Design review of the part built by this model. Coordinates are the model's own, in mm. A direction names the side the tool comes from. Give positions to 0.01 mm unless a question says otherwise; leave off trailing zeros. Write each loop counter-clockwise with the first axis right and the second up, starting at its lowest first coordinate (ties: lowest second). Pieces come first, ordered by that corner, then holes. Notation, with made-up numbers: M 76.25,27 L 118.25,27 A11 ccw 118.25,36 Z; hole C 32,47.25 d5. An arc over 180 degrees is marked long. Answer in a Markdown table with one row per item.
Autodesk Inventor part; units mm, degrees
ref_plane "YZ Plane" through (0, 0, 0) normal (1, 0, 0) x (0, 1, 0)
ref_plane "XZ Plane" through (0, 0, 0) normal (0, 1, 0) x (-1, 0, 0)
ref_plane "XY Plane" through (0, 0, 0) normal (0, 0, 1) x (1, 0, 0)
sketch "スケッチ1" plane through (0, 0, 0) normal (0, 1, 0) x (-1, 0, 0)
  line L0 (0, 0) -> (0, 28.5) construction
  line L1 (0, 30) -> (-7.1789, 30)
  line L2 (-8.2396, 29.5607) -> (-18.0607, 19.7396)
  line L3 (-18.5, 18.6789) -> (-18.5, 0)
  line L4 (-18.5, 0) -> (-17, 0)
  line L5 (-17, 0) -> (-17, 18.6789)
  line L6 (-17, 18.6789) -> (-7.1789, 28.5)
  line L7 (-7.1789, 28.5) -> (0, 28.5)
  line L8 (0, 28.5) -> (0, 30)
  line L9 (0, 0) -> (-17, 0) construction
  line L10 (0, 14.25) -> (-10.7145, 24.9645) construction
  arc A0 (-7.1789, 30) -> (-8.2396, 29.5607) centre (-7.1789, 28.5) ccw
  arc A1 (-18.0607, 19.7396) -> (-18.5, 18.6789) centre (-17, 18.6789) ccw
  dimension "d0" = 28.5
  dimension "d1" = 1.5
  dimension "d2" = 1.5
  dimension "d3" = 135
  dimension "d4" = 1.5
  dimension "d5" = 34
  dimension "d7" = 5
  dimension "d8" = 1.5
extrude "押し出し1" add sketch "スケッチ1" against normal blind 15
sketch "スケッチ2" plane through (17, 0, 0) normal (-1, 0, 0) x (0, 0, 1)
  circle A0 centre (3.25, 4.25) radius 1.3
  arc A1 (4.8202, 7.0955) -> (0, 4.25) centre (3.25, 4.25) ccw
  line L0 (0, 4.25) -> (0, 0)
  line L1 (4.8202, 7.0955) -> (17.6789, 0)
  line L2 (18.6789, 0) -> (0, 0) construction
  line L3 (0, 0) -> (0, -15) construction
  line L4 (0, 0) -> (17.6789, 0)
  line L5 (18.6789, 0) -> (18.6789, -15)
  dimension "d11" = 2.6
  dimension "d12" = 4.25
  dimension "d13" = 3.25
  dimension "d14" = 1
extrude "押し出し2" add sketch "スケッチ2" against normal blind 1.5
sketch "スケッチ3" plane through (7.1789, 0, 28.5) normal (0, 0, -1) x (-1, 0, 0)
  circle A0 centre (1.1789, 8.25) radius 1.3
  line L0 (7.1789, 0) -> (0, 0) construction
  line L1 (7.1789, 0) -> (7.1789, 5.7754) construction
  arc A1 (1.1789, 10.75) -> (-0.5888, 6.4822) centre (1.1789, 8.25) ccw
  line L2 (-0.5888, 6.4822) -> (1.1789, 4.7145)
  line L3 (1.1789, 4.7145) -> (1.1789, 0)
  line L4 (1.1789, 10.75) -> (7.1789, 10.75)
  line L5 (7.1789, 10.75) -> (7.1789, 0)
  line L6 (1.1789, 0) -> (7.1789, 0)
  dimension "d17" = 8.25
  dimension "d18" = 12
  dimension "d19" = 2.6
  dimension "d20" = 2.5
  dimension "d21" = 45
  dimension "d22" = 12
extrude "押し出し3" add sketch "スケッチ3" against normal blind 1.5
sketch "スケッチ4" plane through (18.5, -15, 18.6789) normal (1, 0, 0) x (0, 0, -1)
  line L0 (6, 0) -> (18.6789, 5)
  line L1 (18.6789, 0) -> (18.6789, 19.25) construction
  line L2 (18.6789, 0) -> (18.6789, 5)
  line L3 (0, 0) -> (18.6789, 0) construction
  line L4 (18.6789, 0) -> (6, 0)
  line L5 (0, 15) -> (0, 0) construction
  circle A0 centre (13.1789, 8) radius 1.5
  circle A1 centre (6.1789, 8) radius 1.5
  arc A2 (14.2789, 7.4063) -> (14.2789, 8.5937) centre (13.1789, 8) ccw
  arc A3 (7.2789, 7.4063) -> (7.2789, 8.5937) centre (6.1789, 8) ccw
  dimension "d25" = 5
  dimension "d26" = 6
  dimension "d36" = 3
extrude "押し出し4" cut sketch "スケッチ4" against normal blind 1.5
fillet "フィレット1" radius 2 3 edges at (17.75, -10, 0) (17.75, -15, 12.6789) (6, 4.7145, 29.25)
fillet "フィレット2" radius 1 2 edges at (17.75, 0, 17.6789) (6, 0, 29.25)
sketch "スケッチ5" plane through (8.2396, -15, 29.5607) normal (0.7071, 0, 0.7071) x (0.7071, 0, -0.7071)
  circle A0 centre (6.8, 11) radius 1.5
  circle A1 centre (6.8, 3.6) radius 1.5
  line L0 (0, 15) -> (13.8891, 15)
  line L1 (6.8, 90.0103) -> (6.8, -102.5616) construction
  point P0 (15.0763, 15)
  dimension "d31" = 7.4
  dimension "d32" = 3
  dimension "d33" = 4
extrude "押し出し5" cut sketch "スケッチ5" against normal blind 1.5
mirror "ミラー3" about plane through (0, 0, 0) normal (1, 0, 0) of "押し出し1", "押し出し2", "押し出し3", "押し出し4", "フィレット1", "フィレット2", "押し出し5"
sketch "スケッチ7" plane through (7.1789, -15, 30) normal (0, 0, 1) x (1, 0, 0)
  circle A0 centre (-7.1789, 8) radius 1.5
  arc A1 (-7.8848, 9.0316) -> (-7.8848, 6.9684) centre (-7.1789, 8) ccw
  point P0 (-7.1789, 15)
  dimension "d37" = 3
extrude "押し出し6" cut sketch "スケッチ7" against normal blind 1.5
properties part number "16_024_LOAD_CELL_MOUNT_BRACKET_R1" material "アルミニウム 6061"
1) Add section D-D (y = -4.75). Write out the cut boundary in (x, z).
Geometry says:
| item | result |
|---|---|
| outline | M -18.5,0 L -17,0 L -17,18.68 L -12.91,22.77 L -13.97,23.83 L -18.06,19.74 A1.5 ccw -18.5,18.68 Z; M -12.13,25.67 L -11.07,24.61 L -7.18,28.5 L 7.18,28.5 L 11.07,24.61 L 12.13,25.67 L 8.24,29.56 A1.5 ccw 7.18,30 L -7.18,30 A1.5 ccw -8.24,29.56 Z; M 12.91,22.77 L 17,18.68 L 17,0 L 18.5,0 L 18.5,18.68 A1.5 ccw 18.06,19.74 L 13.97,23.83 Z |
2) Insertion check: P1, Ø5, axis at x = -3, y = -3.5, coming from the -Z side; P2, Ø2.5, axis at y = 4.25, z = 3.25, coming from the -X side; P3, Ø1.6, axis at y = 2, z = 29, coming from the +X side; P4, Ø10, axis at x = -15, y = -11, coming from the +Z side. Each pin has a flat end and moves straight along its axis. Give the tip position at first contact, or say it passes through.
Geometry says:
| item | result |
|---|---|
| P1 | z = 28.5 |
| P2 | through |
| P3 | x = 6 |
| P4 | z = 27.8 |
3) The part is to be moulded in two halves that separate along Z. For faces 4 (the face through (-11.7, -10.5, 25.1)), 5 (the face through (-18, -2, 0)), 6 (the face through (7.185, 5.9, 29.24)), say which applies: released by +Z, released by -Z, zero draft, split by the parting line, or undercut.
Geometry says:
| item | result |
|---|---|
| face 4 | undercut |
| face 5 | released by -Z |
| face 6 | zero draft |
4) Add section B-B (z = 7.75). Write out the cut boundary in (x, y), and give its area (3 significant figures).
Geometry says:
| item | result |
|---|---|
| outline | M -18.5,-13.06 L -17,-13.06 L -17,5.48 L -18.5,5.48 Z; M 17,-13.06 L 18.5,-13.06 L 18.5,5.48 L 17,5.48 Z |
| area | 55.6 mm^2 |
5) Add section A-A (x = 0). Write out the cut boundary in (y, z), and give its area (3 significant figures).
Geometry says:
| item | result |
|---|---|
| outline | M -15,28.5 L -8.5,28.5 L -8.5,30 L -15,30 Z; M -5.5,28.5 L 10.75,28.5 L 10.75,30 L -5.5,30 Z |
| area | 34.1 mm^2 |
6) Add section C-C (z = 3.25). Write out the cut boundary in (x, y), and give its area (3 significant figures).
Geometry says:
| item | result |
|---|---|
| outline | M -18.5,-11.28 L -17,-11.28 L -17,2.95 L -18.5,2.95 Z; M -18.5,5.55 L -17,5.55 L -17,7.5 L -18.5,7.5 Z; M 17,-11.28 L 18.5,-11.28 L 18.5,2.95 L 17,2.95 Z; M 17,5.55 L 18.5,5.55 L 18.5,7.5 L 17,7.5 Z |
| area | 48.5 mm^2 |
7) To check wall thickness, follow probe 1 along X at (y, z) = (-1.5, 6.75); probe 2 along Y at (x, z) = (-17.75, 3.25); probe 3 along Z at (x, y) = (-4, -7.5). State the ranges of each line that lie inside material, in increasing order. Write a range as [from, to].
Geometry says:
| item | result |
|---|---|
| probe 1 | [-18.5, -17], [17, 18.5] |
| probe 2 | [-11.28, 2.95], [5.55, 7.5] |
| probe 3 | [28.5, 30] |
8) For faces 1 (the face through (6.285, 0.301, 29.26)), 2 (the face through (-17, -4, 9)), 3 (the face through (-6.301, 0.285, 29.26)), list the 3-axis set-ups (+Z, -Z, +X, -X, +Y, -Y) from which the entire face can be reached by the end or side of a thin tool; tool diameter is ignored.
Geometry says:
| item | result |
|---|---|
| face 1 | +Z, -Z, +X |
| face 2 | -Z, +Y, -Y |
| face 3 | +Z, -Z, -X |
